The figure shows three views and two pictorial views of one solid part (mm, origin at its lowest corner). Answer the questions. A direction names the side the tool comes from. Round coordinates to 2 decimals unless told otherwise and drop trailing zeros. Order: outer loops, then holes, each group sorted by start corner. A loop starts at its lowest first (then second) coordinate and runs counter-clockwise, first axis right, second up.
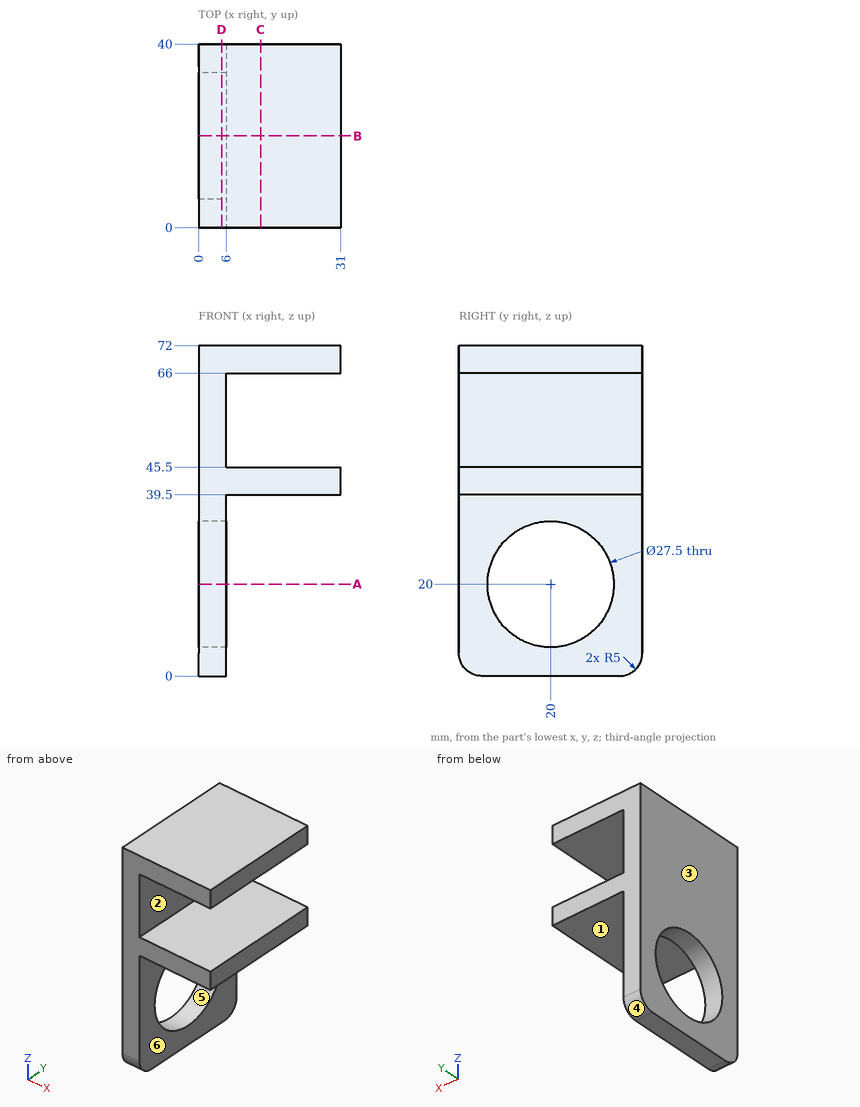
Item 1: Given pin 1 (16.5 mm diameter, centred on y = 24.5, z = 55, fed in from +X); pin 2 (7.5 mm diameter, centred on x = 20.5, y = 11.5, fed in from -Z), each flat-ended and moving along its own axis, determine where each tip first touches the part or whether it passes through.
Item 2: A tool of negligible diameter and unlimited length cuts with its end or side. For the marked faces 1, 2 and 3, from which of +Z, -Z, +X, -X, +Y, -Y can it reach the whole face along a straight path? Write none if from no direction.
Item 3: Find section C-C (x = 13.5). Write down the section's boundary in (y, z), plus the area to 3 significant figures.
Item 4: For a pull along Y with two mould halves and no side action, classify the marked faces 4, 5 and 6 as released by +Y, released by -Y, zero draft, split by the parting line, or undercut.
Item 5: Find section A-A (z = 20). Write down the section's boundary in (x, y), plus the area to 3 significant figures.
Item 6: Find section D-D (x = 5). Write down the section's boundary in (y, z), plus the area to 3 significant figures.
Item 7: Find the intervals of material crossed by line 1 along Z through (x, y) = (2.6, 20); line 2 along Z through (x, y) = (20.5, 2.5); line 3 along X through (y, z) = (21, 36), in increasing order.
Item 8: Find section B-B (y = 20). Write down the section's boundary in (x, z), plus the area to 3 significant figures.
Model answer:
1. pin 1: stops at x = 6
1. pin 2: stops at z = 39.5
2. face 1: -Z, +X, +Y, -Y
2. face 2: +X, +Y, -Y
2. face 3: +Z, -Z, -X, +Y, -Y
3. outline: (0, 39.5) - (40, 39.5) - (40, 45.5) - (0, 45.5) - close; (0, 66) - (40, 66) - (40, 72) - (0, 72) - close
3. area: 480 mm2
4. face 4: released by +Y
4. face 5: undercut
4. face 6: zero draft
5. outline: (0, 0) - (6, 0) - (6, 6.25) - (0, 6.25) - close; (0, 33.75) - (6, 33.75) - (6, 40) - (0, 40) - close
5. area: 75.0 mm2
6. outline: (0, 5) arc R5 ccw to (5, 0) - (35, 0) arc R5 ccw to (40, 5) - (40, 72) - (0, 72) - close; hole circle Ø27.5 at (20, 20)
6. area: 2,280 mm2
7. line 1: z = 0 to 6.25, 33.75 to 72
7. line 2: z = 39.5 to 45.5, 66 to 72
7. line 3: x = 0 to 6
8. outline: (0, 0) - (6, 0) - (6, 6.25) - (0, 6.25) - close; (0, 33.75) - (6, 33.75) - (6, 39.5) - (31, 39.5) - (31, 45.5) - (6, 45.5) - (6, 66) - (31, 66) - (31, 72) - (0, 72) - close
8. area: 567 mm2
